```python
from build123d import *

# Parameters (mm, degrees)
F0_W     = 160
F0_H     = 120
F0_R     = 1.85
F0_R_2   = 2.5
F0_W_2   = 12.5
F0_H_2   = 19.5
F0_W_3   = 11
F0_H_3   = 24
F1_DEPTH = 3
F2_W     = 160
F2_H     = 120
F2_W_2   = 154
F2_H_2   = 114
F3_DEPTH = 75
F5_DEPTH = 160.001
F6_W     = 10
F6_H     = 99.564
F6_R     = 1.5
F7_DEPTH = 3


with BuildPart() as f1:
    # F0 (on Front) → F1 (new body)
    with BuildSketch(Plane.XZ):
        Rectangle(F0_W, F0_H)
        with Locations((60, -41.5)):
            Circle(F0_R, mode=Mode.SUBTRACT)
        with Locations((-59.2675954103, 0)):
            Circle(F0_R_2, mode=Mode.SUBTRACT)
        with Locations((-32, 0)):
            Rectangle(F0_W_2, F0_H_2, mode=Mode.SUBTRACT)
        with Locations((-9, 0)):
            Rectangle(F0_W_2, F0_H_2, mode=Mode.SUBTRACT)
        with Locations((14, 0)):
            Rectangle(F0_W_2, F0_H_2, mode=Mode.SUBTRACT)
        with Locations((37, 0)):
            Rectangle(F0_W_2, F0_H_2, mode=Mode.SUBTRACT)
        with Locations((60, 0)):
            Rectangle(F0_W_3, F0_H_3, mode=Mode.SUBTRACT)
        with Locations((60, 41.5)):
            Circle(F0_R, mode=Mode.SUBTRACT)
    extrude(amount=F1_DEPTH)

    # F2 (on face) → F3 (join)
    with BuildSketch(Plane(origin=(0, 0, 0), x_dir=(-1, 0, 0), z_dir=(0, 1, 0))):
        Rectangle(F2_W, F2_H)
        Rectangle(F2_W_2, F2_H_2, mode=Mode.SUBTRACT)
    extrude(amount=F3_DEPTH)

    # F4 (on face) → F5 (cut, through all)
    with BuildSketch(Plane.YZ.offset(80)):
        Polygon((75, 60), (5.7179676972, 60), (55.5, -26.2250092524), (-3, -60), (75, -60), align=None)
    extrude(amount=-F5_DEPTH, mode=Mode.SUBTRACT)

    # F6 (on face) → F7 (join)
    with BuildSketch(Plane(origin=(0, 30.2692378865, 17.4759526419), x_dir=(-1, 0, 0), z_dir=(0, 0.8660254038, 0.5))):
        with Locations((-82, -0.6795242271)):
            Rectangle(F6_W, F6_H)
        with Locations((-84, -37.7615242271)):
            Circle(F6_R, mode=Mode.SUBTRACT)
        with Locations((-84, -0.6795242271)):
            Circle(F6_R, mode=Mode.SUBTRACT)
        with Locations((-84, 36.4024757729)):
            Circle(F6_R, mode=Mode.SUBTRACT)
        with Locations((82, -0.6795242271)):
            Rectangle(F6_W, F6_H)
        with Locations((84, -37.7615242271)):
            Circle(F6_R, mode=Mode.SUBTRACT)
        with Locations((84, -0.6795242271)):
            Circle(F6_R, mode=Mode.SUBTRACT)
        with Locations((84, 36.4024757729)):
            Circle(F6_R, mode=Mode.SUBTRACT)
    extrude(amount=F7_DEPTH)


solid = f1.part
```
Verification items for the finished model (mm, model axes). A direction names the side the tool comes from. Round coordinates to 2 decimals unless told otherwise and drop trailing zeros. Write each loop counter-clockwise with the first axis right and the second up, starting at its lowest first coordinate (ties: lowest second). Pieces come first, ordered by that corner, then holes. Notation, with made-up numbers: (52, -26.75) - (106, -26.75) arc R13 ccw to (106, -12.75) - close; hole circle Ø3 at (-30, 15.25). An arc over 180 degrees is marked (long way). Answer as a JSON object with one key per item and string values. Group by question number.
Q1. Section check A-A, the plane x = 60. Enter the section's corners in (y, z).
Q2. Mould release check, pull along Z, two halves, no side actions. Record for faces 1 (the flat face through (-81.9, 30.26, 17.49)), 2 (the flat face through (80, 19, -1)), 3 (the cylindrical face through (-85.43, 31.66, 18.02)): released by +Z, released by -Z, zero draft, split by the parting line, or undercut.
Q3. Tool access check on faces 4 (the flat face through (81.99, 30.26, 17.49)), 5 (the flat face through (1, 4, 57)), 6 (the flat face through (-80, 19, -1)). Record the directions out of +Z, -Z, +X, -X, +Y, -Y that give a thin tool (end or side, any length) a straight path to the whole face; none if there is none.
Q4. Section check C-C, the plane z = -41.5. Enter the section's corners in (x, y).
Q5. Go/stop test with flat-tipped pins: pin 1 Ø1.8 at (x, y) = (-8, 0.5) entering from +Z; pin 2 Ø3.5 at (x, y) = (13, -1.5) entering from -Z; pin 3 Ø6 at (x, z) = (60, -41.5) entering from +Y; pin 4 Ø8 at (x, z) = (15.5, 3) entering from +Y. Record where each tip stops, or that it passes through.
Q6. Thickness scan on line 1 (X direction, y = 26, z = -8); line 2 (Y direction, x = -8.5, z = -22.5); line 3 (X direction, y = -2, z = 41). Record the ranges inside material, lowest first.
Q7. Section check B-B, the plane y = 36.5. Enter the section's corners in (x, z).
Q8. Section check D-D, the plane x = -42. Enter the section's corners in (y, z).
Found:
{
 "1": {"outline": "(-3, -60) - (2.2, -57) - (0, -57) - (0, -43.35) - (-3, -43.35) - close; (-3, -39.65) - (0, -39.65) - (0, -12) - (-3, -12) - close; (-3, 12) - (0, 12) - (0, 39.65) - (-3, 39.65) - close; (-3, 43.35) - (0, 43.35) - (0, 57) - (7.45, 57) - (5.72, 60) - (-3, 60) - close"},
 "2": {"face 1": "released by -Z", "face 2": "zero draft", "face 3": "undercut"},
 "3": {"face 4": "-Z, +X, -Y", "face 5": "+Y", "face 6": "-Z, -X, -Y"},
 "4": {"outline": "(-80, -3) - (58.15, -3) - (58.15, 0) - (-77, 0) - (-77, 29.04) - (-80, 29.04) - close; (61.85, -3) - (80, -3) - (80, 29.04) - (77, 29.04) - (77, 0) - (61.85, 0) - close"},
 "5": {"pin 1": "stops at z = 60", "pin 2": "stops at z = -60", "pin 3": "stops at y = 0", "pin 4": "passes through"},
 "6": {"line 1": "x = -80 to -77, 77 to 80", "line 2": "y = -3 to 0", "line 3": "x = -80 to 58.22, 61.78 to 80"},
 "7": {"outline": "(-87, 6.68) - (-80, 6.68) - (-80, -37.19) - (-77, -37.19) - (-77, 12.68) - (-87, 12.68) - close; (77, -37.19) - (80, -37.19) - (80, 6.68) - (87, 6.68) - (87, 12.68) - (77, 12.68) - close"},
 "8": {"outline": "(-3, -60) - (2.2, -57) - (0, -57) - (0, 57) - (7.45, 57) - (5.72, 60) - (-3, 60) - close"}
}
